Autodesk Inventor part; units mm, degrees
ref_plane "YZ Plane" through (0, 0, 0) normal (1, 0, 0) x (0, 1, 0)
ref_plane "XZ Plane" through (0, 0, 0) normal (0, 1, 0) x (-1, 0, 0)
ref_plane "XY Plane" through (0, 0, 0) normal (0, 0, 1) x (1, 0, 0)
sketch "Sketch1" plane through (0, 0, 0) normal (0, 1, 0) x (-1, 0, 0)
  circle A0 centre (4.6155, 11.5612) radius 26.0349
  point P0 (0, 0)
extrude "Extrusion1" add sketch "Sketch1" along normal blind 25.4
sketch "Sketch2" plane through (-4.6155, 25.4, 11.5612) normal (0, 1, 0) x (1, 0, 0)
  line L0 (-9.602, 3.1232) -> (-33.7988, 42.4236)
  line L1 (-33.7988, 42.4236) -> (11.6664, 78.0251)
  arc A0 (24.8436, 79.6434) -> (11.6664, 78.0251) centre (19.5984, 67.8956) ccw
  line L2 (24.8436, 79.6434) -> (39.9619, 55.0882)
  arc A1 (39.4079, 50.3607) -> (39.9619, 55.0882) centre (36.6923, 53.0751) ccw
  line L3 (39.4079, 50.3607) -> (21.8383, 37.6459)
  arc A2 (21.8383, 37.6459) -> (12.1988, 45.3621) centre (3.0409, 24.0425) ccw
  line L4 (12.1988, 45.3621) -> (3.0438, 49.2947)
  arc A3 (3.0438, 49.2947) -> (-3.6684, 48.7425) centre (0.208, 42.6931) ccw
  line L5 (-3.6684, 48.7425) -> (-11.7064, 40.2083)
  arc A4 (-11.7064, 40.2083) -> (-2.2121, 18.2269) centre (-2.2136, 31.2674) ccw
  line L6 (-2.2121, 18.2269) -> (32.4028, 9.4421)
  line L7 (32.4028, 9.4421) -> (13.4408, -10.6903)
  line L8 (13.4408, -10.6903) -> (-9.602, 3.1232)
  point P0 (4.6155, 11.5612)
extrude "Extrusion2" add sketch "Sketch2" along normal blind 25.4
properties part number "Test part"
Geometry: final body of the model. Coordinates: model frame, mm. A direction names the side the tool comes from. Round coordinates to 2 decimals unless told otherwise and drop trailing zeros. Order: outer loops, then holes, each group sorted by start corner. A loop starts at its lowest first (then second) coordinate and runs counter-clockwise, first axis right, second up. Notation, with made-up numbers: (58, 5.25) -> (83, 5.25) arc R23 cw to (83, 32.25) -> close; hole circle Ø8 at (-5, 78.5). An arc over 180 degrees is marked (long way). Use one line per item in the form item = value. Start each with the question number.
1. Pin query (flat end, axial travel): pin 1 Ø4 at (y, z) = (25, 25.5) entering from -X; pin 2 Ø2 at (y, z) = (27.5, -35) entering from +X; pin 3 Ø6 at (x, y) = (-24.5, 30) entering from -Z. Return the tip coordinate at first contact, or that it passes through.
2. Cut plane A-A (y = 28.5). Return the cut outline in (x, z).
3. Reachability of faces 1 (the face through (-2.535, 37.922, 15.441)), 2 (the face through (1, 25.4, -9)), 3 (the face through (26.13, 37.92, -32.53)) from +Z, -Z, +X, -X, +Y, -Y: full face, straight path, thin tool, end or side. Return the list, or none.
4. Cut plane D-D (x = 4.5). Return the cut outline in (y, z), then the cut area to 3 significant figures.
5. Draft query along Z for faces 4 (the face through (18.439, 37.922, 12.044)), 5 (the face through (-2, 25.4, -45)), 6 (the face through (-5.05, 37.92, -38.29)). Return one class per face: pulls with the +Z half, pulls with the -Z half, needs draft (parallel to the pull), parting line crosses it, or undercut.
6. Cut plane B-B (x = 12). Return the cut outline in (y, z), then the cut area to 3 significant figures.
7. Cut plane C-C (z = 7). Return the cut outline in (x, y).
8. Line query: probe 1 along Z at (x, y) = (-4, 29); probe 2 along Y at (x, z) = (-28, 20.5); probe 3 along Z at (x, y) = (27, 32.5) (3 decimals). Output: solid intervals per line, ascending.
Solution:
q1.pin_1 = -27.75
q1.pin_2 = 30.92
q1.pin_3 = -44.11
q2.outline = (-38.41, -30.86) -> (7.05, -66.46) arc R12.87 ccw to (20.23, -68.08) -> (35.35, -43.53) arc R3.84 ccw to (34.79, -38.8) -> (17.22, -26.08) arc R23.2 cw to (7.58, -33.8) -> (-1.57, -37.73) arc R7.18 cw to (-8.28, -37.18) -> (-16.32, -28.65) arc R13.04 cw to (-6.83, -6.67) -> (27.79, 2.12) -> (8.83, 22.25) -> (-14.22, 8.44) -> close
q3.face_1 = +Z, -X, +Y
q3.face_2 = +X, +Y
q3.face_3 = +X, +Y, -Y
q4.outline = (0, -12.83) -> (25.4, -12.83) -> (25.4, -3.79) -> (50.8, -3.79) -> (50.8, 19.66) -> (25.4, 19.66) -> (25.4, 35.95) -> (0, 35.95) -> close; (25.4, -64.47) -> (50.8, -64.47) -> (50.8, -35.13) -> (25.4, -35.13) -> close
q4.area = 2,580 mm^2
q5.face_4 = pulls with the +Z half
q5.face_5 = needs draft
q5.face_6 = undercut
q6.outline = (0, -8.48) -> (25.4, -8.48) -> (25.4, -1.89) -> (50.8, -1.89) -> (50.8, 18.88) -> (25.4, 18.88) -> (25.4, 31.6) -> (0, 31.6) -> close; (25.4, -68.85) -> (50.8, -68.85) -> (50.8, -31.3) -> (25.4, -31.3) -> close
q6.area = 2,500 mm^2
q7.outline = (-30.25, 0) -> (21.02, 0) -> (21.02, 25.4) -> (23.19, 25.4) -> (23.19, 50.8) -> (-15.1, 50.8) -> (-15.1, 25.4) -> (-30.25, 25.4) -> close
q8.probe_1 = -57.81 to -38.31, -5.95 to 14.56
q8.probe_2 = 0 to 25.4
q8.probe_3 = -57.083 to -33.16, 1.919 to 2.955
